Input: part model. Units: mm. Frame: model coordinates. Face numbers are marked on the shaded views. A direction names the side the tool comes from. Give positions to 0.01 mm unless a question says otherwise; leave off trailing zeros. Write each loop counter-clockwise with the first axis right and the second up, starting at its lowest first coordinate (ties: lowest second). Pieces come first, ordered by that corner, then holes. Notation, with made-up numbers: M 29.25,69 L 59.25,69 A25 cw 59.25,100 Z; hole C 23,-3 d11. An arc over 180 degrees is marked long. Use CSV: the item, a comma, the result in double quotes. Start each with the question number.
from build123d import *

# Parameters (mm, degrees)
SKETCH2_W                = 80
SKETCH2_H                = 80
BOSS_EXTRUDE1_DEPTH      = 10
SKETCH3_R                = 35.3
BOSS_EXTRUDE2_DEPTH      = 9.5
SKETCH5_R                = 29.3
CUT_EXTRUDE1_DEPTH       = 5.3
SKETCH6_R                = 37.5
SKETCH6_R_2              = 33
CUT_EXTRUDE4_DEPTH       = 4
SKETCH8_R                = 26.5
CUT_EXTRUDE10_DEPTH      = 2.5
SKETCH9_R                = 29.3
CUT_EXTRUDE11_DEPTH      = 5.3
SKETCH10_R               = 25
CUT_EXTRUDE12_DEPTH      = 11.3
SKETCH11_R               = 5
CUT_EXTRUDE13_DEPTH      = 64
CUT_EXTRUDE13_DEPTH_BACK = 36.3


with BuildPart() as part:
    # Sketch2 → Boss-Extrude1 (new body)
    with BuildSketch(Plane.XY):
        with Locations((0, 40)):
            Rectangle(SKETCH2_W, SKETCH2_H)
    extrude(amount=BOSS_EXTRUDE1_DEPTH)

    # Sketch3 → Boss-Extrude2 (add)
    with BuildSketch(Plane.XY.offset(10)):
        with Locations((0, 40)):
            Circle(SKETCH3_R)
    extrude(amount=BOSS_EXTRUDE2_DEPTH)

    # Sketch5 → Cut-Extrude1 (cut)
    with BuildSketch(Plane.XY.offset(11.3)):
        with Locations((0, 40)):
            Circle(SKETCH5_R)
    extrude(amount=CUT_EXTRUDE1_DEPTH, mode=Mode.SUBTRACT)

    # Sketch6 → Cut-Extrude4 (cut)
    with BuildSketch(Plane.XY.offset(11.3)):
        with Locations((0, 40)):
            Circle(SKETCH6_R)
        with Locations((0, 40)):
            Circle(SKETCH6_R_2, mode=Mode.SUBTRACT)
    extrude(amount=CUT_EXTRUDE4_DEPTH, mode=Mode.SUBTRACT)

    # Sketch8 → Cut-Extrude10 (cut)
    with BuildSketch(Plane.XY.offset(19.5)):
        with Locations((0, 40)):
            Circle(SKETCH8_R)
    extrude(amount=-CUT_EXTRUDE10_DEPTH, mode=Mode.SUBTRACT)

    # Sketch9 → Cut-Extrude11 (cut)
    with BuildSketch(Plane.XY.offset(17)):
        with Locations((0, 40)):
            Circle(SKETCH9_R)
    extrude(amount=-CUT_EXTRUDE11_DEPTH, mode=Mode.SUBTRACT)

    # Sketch10 → Cut-Extrude12 (cut)
    with BuildSketch(Plane(origin=(0, 0, 0), x_dir=(-1, 0, 0), z_dir=(0, 0, -1))):
        with Locations((0, 40)):
            Circle(SKETCH10_R)
    extrude(amount=-CUT_EXTRUDE12_DEPTH, mode=Mode.SUBTRACT)

    # Sketch11 → Cut-Extrude13 (cut, two sides)
    with BuildSketch(Plane.XY) as cut_extrude13_sk:
        with Locations((-31, 71)):
            Circle(SKETCH11_R)
        with Locations((31, 71)):
            Circle(SKETCH11_R)
        with Locations((31, 9)):
            Circle(SKETCH11_R)
        with Locations((-31, 9)):
            Circle(SKETCH11_R)
    extrude(amount=CUT_EXTRUDE13_DEPTH, mode=Mode.SUBTRACT)
    extrude(cut_extrude13_sk.sketch, amount=-CUT_EXTRUDE13_DEPTH_BACK, mode=Mode.SUBTRACT)


solid = part.part
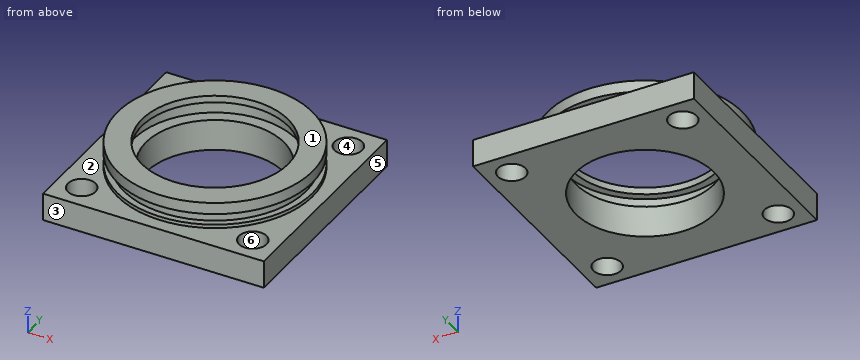
Q1. Section A-A, the plane x = 0. Return the cut outline in (y, z), and give its area (3 significant figures).
Q2. Section D-D, the plane x = 31. Return the cut outline in (y, z), and give its area (3 significant figures).
Q3. First-contact query: pin 1 Ø9 at (x, y) = (31, 71) entering from -Z; pin 2 Ø13 at (x, y) = (-31, 71) entering from +Z. Flat tips, straight axial feed; report the tip coordinate or a pass-through.
Q4. Material intervals for L1, parallel to Y at x = -31, z = 7.25; L2, parallel to X at y = 71, z = 2.75; L3, parallel to Z at x = -21, y = 58, sorted ascending. Write a range as [from, to].
Q5. Section B-B, the plane z = 7. Return the cut outline in (x, y).
Q6. Set-up query: the marked faces 1 and 2. Return all of +Z, -Z, +X, -X, +Y, -Y with unobstructed straight access to the full face (end or side cutting, diameter ignored); none if empty.
Q7. Section C-C, the plane y = 9. Return the cut outline in (x, z), and give its area (3 significant figures).
Q8. Pull-direction query (X, two-part tool) for the marked faces 3, 4, 5 and 6; classes: released by +X, released by -X, zero draft, split by the parting line, or undercut.
Check result:
1,outline,"M 0,0 L 15,0 L 15,11.3 L 10.7,11.3 L 10.7,17 L 13.5,17 L 13.5,19.5 L 4.7,19.5 L 4.7,15.3 L 7,15.3 L 7,11.3 L 4.7,11.3 L 4.7,10 L 0,10 Z; M 65,0 L 80,0 L 80,10 L 75.3,10 L 75.3,11.3 L 73,11.3 L 73,15.3 L 75.3,15.3 L 75.3,19.5 L 66.5,19.5 L 66.5,17 L 69.3,17 L 69.3,11.3 L 65,11.3 Z"
1,area,"421 mm²"
2,outline,"M 0,0 L 4,0 L 4,10 L 0,10 Z; M 14,0 L 66,0 L 66,10 L 56.88,10 L 56.88,11.3 L 51.31,11.3 L 51.31,15.3 L 56.88,15.3 L 56.88,19.5 L 23.12,19.5 L 23.12,15.3 L 28.69,15.3 L 28.69,11.3 L 23.12,11.3 L 23.12,10 L 14,10 Z; M 76,0 L 80,0 L 80,10 L 76,10 Z"
2,area,"876 mm²"
3,pin 1,"passes through"
3,pin 2,"stops at z = 10"
4,L1,"y = [0, 4], [14, 66], [76, 80]"
4,L2,"x = [-40, -36], [-26, 26], [36, 40]"
4,L3,"z = [0, 11.3], [17, 19.5]"
5,outline,"M -40,0 L 40,0 L 40,80 L -40,80 Z; hole C -31,9 d10; hole C -31,71 d10; hole C 0,40 d50; hole C 31,9 d10; hole C 31,71 d10"
6,face 1,"+Z, +X, -X, +Y, -Y"
6,face 2,"+Z"
7,outline,"M -40,0 L -36,0 L -36,10 L -40,10 Z; M -26,0 L 26,0 L 26,10 L 16.88,10 L 16.88,11.3 L 11.31,11.3 L 11.31,15.3 L 16.88,15.3 L 16.88,19.5 L -16.88,19.5 L -16.88,15.3 L -11.31,15.3 L -11.31,11.3 L -16.88,11.3 L -16.88,10 L -26,10 Z; M 36,0 L 40,0 L 40,10 L 36,10 Z"
7,area,"876 mm²"
8,face 3,"zero draft"
8,face 4,"undercut"
8,face 5,"released by +X"
8,face 6,"undercut"
